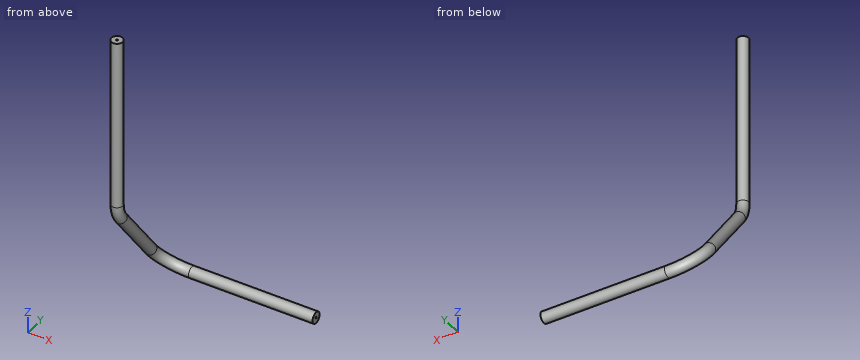
```python
from build123d import *

# Parameters (mm, degrees)
SKICA4_R   = 3
SKICA4_R_2 = 0.5


with BuildPart() as part:
    # Táhnout po křivce1: sweep along a curve in space
    with BuildLine() as t_hnout_po_k_ivce1_path:
        Line((82, 0, 0), (16, 0, 0))
        ThreePointArc((16, 0, 0), (4.686291501, -2.845029331, 3.723860381), (0, -9.713537728, 12.714054617))
        Line((0, -9.713537728, 12.714054617), (0, -34.914054617, 45.699024368))
        ThreePointArc((0, -34.914054617, 45.699024368), (0, -37.35626725, 50.285422244), (0, -38.2, 55.412562096))
        Line((0, -38.2, 55.412562096), (0, -38.2, 147))
    # Skica4 → Táhnout po křivce1 (sweep)
    with BuildSketch(Plane(origin=(82, 0, 0), x_dir=(0, 0, -1), z_dir=(1, 0, 0))):
        Circle(SKICA4_R)
        Circle(SKICA4_R_2, mode=Mode.SUBTRACT)
    sweep(path=t_hnout_po_k_ivce1_path.line)


solid = part.part
```
The model under review builds one solid part; all positions refer to its coordinate system, in mm. Coordinates: 2 decimals unless noted, no trailing zeros. Write each loop counter-clockwise with the first axis right and the second up, starting at its lowest first coordinate (ties: lowest second). Pieces come first, ordered by that corner, then holes.
1) We need section B-B on z = 84. State the section outline as (x, y) points, then the cut area to 3 significant figures.
2) Clearance check with a flat-ended pin moving along its axis: pin 1 Ø12 at (x, z) = (10, 132) entering from -Y. State where the tip first meets the part, or that it passes through.
3) We need section A-A on x = 67. State the section outline as (y, z) points.
4) To check wall thickness, follow probe 1 along Y at (x, z) = (61, 0); probe 2 along X at (y, z) = (-8.5, 11.5) (3 decimals). State the ranges of each line that lie inside material, in increasing order.
Answer list:
1. outline: circle Ø6 at (0, -38.2); hole circle Ø1 at (0, -38.2)
1. area: 27.5 mm2
2. pin 1: passes through
3. outline: circle Ø6 at (0, 0); hole circle Ø1 at (0, 0)
4. probe 1: y = -3 to -0.5, 0.5 to 3
4. probe 2: x = -2.915 to -0.357, 0.539 to 3.103
